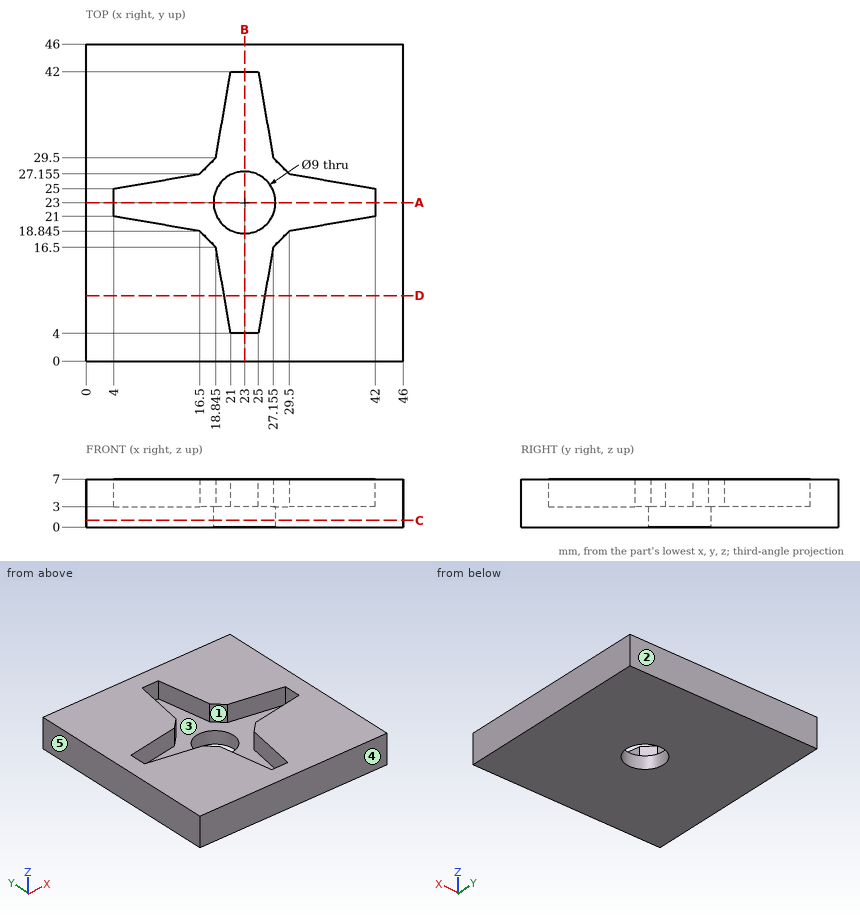
Check sheet for the drawn part. Datum: minimum x, y, z corner. Units: mm. A direction names the side the tool comes from. Coordinates: 2 decimals unless noted, no trailing zeros. Loops run counter-clockwise (first coordinate to the right, second up) from the corner with the lowest first, then second, coordinate; pieces in that order, holes last. Notation, with made-up numbers: (-4.75, 73.25) - (25.25, 73.25) arc R15 cw to (25.25, 84.25) - close; hole circle Ø4 at (72, -31.5). An arc over 180 degrees is marked (long way). Put each result on its own line as item: value.
Item 1: Section check D-D (y = 9.5). Enter the section's corners in (x, z), then the cut area to 3 significant figures.
Conclusion:
outline: (0, 0) - (46, 0) - (46, 7) - (25.95, 7) - (25.95, 3) - (20.05, 3) - (20.05, 7) - (0, 7) - close
area: 298 mm2
Item 2: Gauge pin test, flat ends, axial feed: pin 1 Ø4 at (x, y) = (16.5, 23) entering from +Z; pin 2 Ø7 at (x, y) = (23, 23) entering from -Z. Record the tip position at first contact, or that the pin passes through.
Conclusion:
pin 1: stops at z = 3
pin 2: passes through
Item 3: Scan lines: line 1 along Y through (x, z) = (21.5, 4.5); line 2 along Y through (x, z) = (23, 1.85); line 3 along Z through (x, y) = (21, 36). Record each from-to range of solid material in increasing order.
Conclusion:
line 1: y = 0 to 4, 42 to 46
line 2: y = 0 to 18.5, 27.5 to 46
line 3: z = 0 to 3
Item 4: Set-up check for the marked faces 1 and 2: record each of +Z, -Z, +X, -X, +Y, -Y from which the full face is reachable in a straight line by a thin tool's end or side.
Conclusion:
face 1: +Z
face 2: +Z, -Z, +X, -X, +Y
Item 5: Draft check along X on the marked faces 3, 4 and 5. Enter one of: pulls with the +X half, pulls with the -X half, needs draft (parallel to the pull), parting line crosses it, or undercut.
Conclusion:
face 3: undercut
face 4: needs draft
face 5: pulls with the -X half
Item 6: Section check A-A (y = 23). Enter the section's corners in (x, z).
Conclusion:
outline: (0, 0) - (18.5, 0) - (18.5, 3) - (4, 3) - (4, 7) - (0, 7) - close; (27.5, 0) - (46, 0) - (46, 7) - (42, 7) - (42, 3) - (27.5, 3) - close
Item 7: Section check C-C (z = 1). Enter the section's corners in (x, y).
Conclusion:
outline: (0, 0) - (46, 0) - (46, 46) - (0, 46) - close; hole circle Ø9 at (23, 23)
